Geometry: see drawing. Coordinates: mm, zero at the bounding-box minimum. A direction names the side the tool comes from. Give positions to 0.01 mm unless a question says otherwise; leave off trailing zeros. Loops run counter-clockwise (first coordinate to the right, second up) from the corner with the lowest first, then second, coordinate; pieces in that order, holes last. Notation, with made-up numbers: (69, 0.5) -> (96, 0.5) arc R16 ccw to (96, 8.5) -> close; hole circle Ø10 at (-25, -31). An arc over 180 degrees is marked (long way). Use CSV: the item, a comma, the result in double quotes.
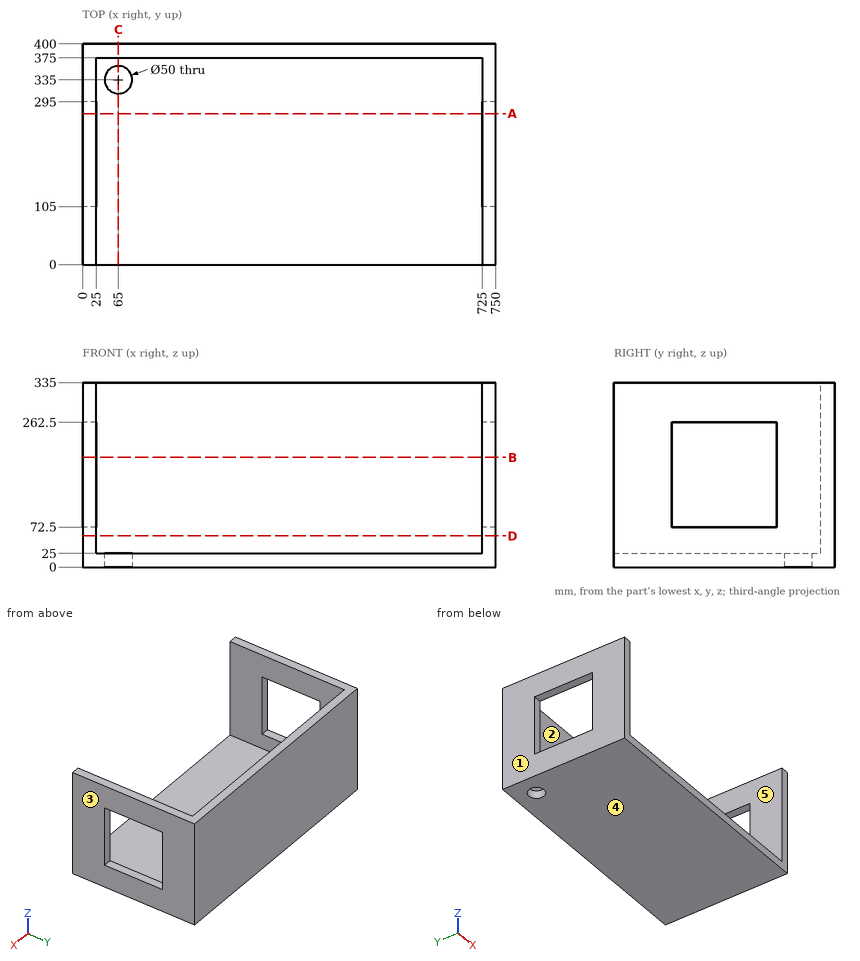
1) Reachability of the marked faces 1 and 2 from +Z, -Z, +X, -X, +Y, -Y: full face, straight path, thin tool, end or side. Return the list, or none.
From the geometry:
face 1,"+Z, -Z, -X, +Y, -Y"
face 2,"+Z, -Y"
2) Mould query, pull axis X, two halves, no side actions, for the marked faces 3, 4 and 5. Classes: pulls with the +X half, pulls with the -X half, needs draft (parallel to the pull), parting line crosses it, or undercut.
From the geometry:
face 3,"pulls with the +X half"
face 4,"needs draft"
face 5,"undercut"
3) Contact query for flat-ended pins moving along their axis: pin 1 (4 mm diameter, centred on x = 473.5, z = 85, fed in from -Y); pin 2 (2 mm diameter, centred on x = 177.5, y = 103.5, fed in from +Z). Output: stop coordinate, or through.
From the geometry:
pin 1,"stops at y = 375"
pin 2,"stops at z = 25"
4) Section query C-C (x = 65). Return loops of the section in (y, z), then the cut area to 3 significant figures.
From the geometry:
outline,"(0, 0) -> (310, 0) -> (310, 25) -> (0, 25) -> close; (360, 0) -> (400, 0) -> (400, 335) -> (375, 335) -> (375, 25) -> (360, 25) -> close"
area,"16,500 mm^2"
5) Section query D-D (z = 57). Return loops of the section in (x, y), then the cut area to 3 significant figures.
From the geometry:
outline,"(0, 0) -> (25, 0) -> (25, 375) -> (725, 375) -> (725, 0) -> (750, 0) -> (750, 400) -> (0, 400) -> close"
area,"37,500 mm^2"
6) Ray query, line 1 (X direction, y = 68, z = 45); line 2 (Y direction, x = 65, z = 7); line 3 (Z direction, x = 153, y = 33). Return the intervals inside material, ascending.
From the geometry:
line 1,"x = 0 to 25, 725 to 750"
line 2,"y = 0 to 310, 360 to 400"
line 3,"z = 0 to 25"
7) Section query B-B (z = 199). Return loops of the section in (x, y), then the cut area to 3 significant figures.
From the geometry:
outline,"(0, 0) -> (25, 0) -> (25, 105) -> (0, 105) -> close; (0, 295) -> (25, 295) -> (25, 375) -> (725, 375) -> (725, 295) -> (750, 295) -> (750, 400) -> (0, 400) -> close; (725, 0) -> (750, 0) -> (750, 105) -> (725, 105) -> close"
area,"28,000 mm^2"
8) Section query A-A (y = 273.5). Return loops of the section in (x, z), then the cut area to 4 significant figures.
From the geometry:
outline,"(0, 0) -> (750, 0) -> (750, 72.5) -> (725, 72.5) -> (725, 25) -> (25, 25) -> (25, 72.5) -> (0, 72.5) -> close; (0, 262.5) -> (25, 262.5) -> (25, 335) -> (0, 335) -> close; (725, 262.5) -> (750, 262.5) -> (750, 335) -> (725, 335) -> close"
area,"24,750 mm^2"
